Autodesk Inventor part; units mm, degrees
ref_plane "YZ Plane" through (0, 0, 0) normal (1, 0, 0) x (0, 1, 0)
ref_plane "XZ Plane" through (0, 0, 0) normal (0, 1, 0) x (-1, 0, 0)
ref_plane "XY Plane" through (0, 0, 0) normal (0, 0, 1) x (1, 0, 0)
sketch "Sketch1" plane through (0, 0, 0) normal (0, 0, 1) x (1, 0, 0)
  line L0 (-47.5, -14) -> (47.5, -14)
  line L1 (47.5, -14) -> (47.5, 14)
  line L2 (47.5, 14) -> (-47.5, 14)
  line L3 (-47.5, 14) -> (-47.5, -14)
  line L4 (-47.5, -14) -> (47.5, 14) construction
  line L5 (47.5, -14) -> (-47.5, 14) construction
  line L6 (47.5, 14) -> (61.5, 14)
  line L7 (61.5, 14) -> (61.5, -14)
  line L8 (61.5, -14) -> (47.5, -14)
  line L9 (47.5, -14) -> (47.5, 14)
  point P0 (0, 0)
  dimension "d0" = 95
  dimension "d1" = 28
  dimension "d2" = 14
  dimension "d3" = 28
extrude "Extrusion1" add sketch "Sketch1" along normal blind 14
sketch "Sketch2" plane through (0, 0, 14) normal (0, 0, 1) x (1, 0, 0)
  circle A0 centre (47.5, 0) radius 5
  line L0 (61.5, -14) -> (61.5, 14)
  line L1 (-47.5, -14) -> (61.5, -14)
  point P0 (0, 0)
  dimension "d6" = 10
  dimension "d7" = 14
  dimension "d8" = 14
extrude "Extrusion2" cut sketch "Sketch2" against normal blind 14
sketch "Sketch3" plane through (-47.5, -14, 0) normal (-1, 0, 0) x (0, 0, 1)
  circle A0 centre (7, 14) radius 5
  line L0 (0, 28) -> (14, 28)
  line L1 (14, 28) -> (14, 0)
  circle A1 centre (7, 14) radius 25
  point P0 (0, 14)
  dimension "d11" = 10
  dimension "d12" = 14
  dimension "d13" = 7
  dimension "d14" = 50
extrude "Extrusion3" cut sketch "Sketch3" against normal blind 52
properties part number "MSAL Pushing Thing"
Could you check a few things on this model? Use its own coordinates, in mm. Round coordinates to 2 decimals unless told otherwise and drop trailing zeros. Write each loop counter-clockwise with the first axis right and the second up, starting at its lowest first coordinate (ties: lowest second). Pieces come first, ordered by that corner, then holes. Notation, with made-up numbers: (-27, 41.5) -> (-12, 41.5) arc R7 cw to (-12, 50.5) -> close; hole circle Ø9 at (-10.75, 20). An arc over 180 degrees is marked (long way). Use a Markdown table: item, result.
1. If we section it at B-B (x = 47.5): List the corners of the cut face in (y, z) for me.
Answer key:
| item | result |
|---|---|
| outline | (-14, 0) -> (-5, 0) -> (-5, 14) -> (-14, 14) -> close; (5, 0) -> (14, 0) -> (14, 14) -> (5, 14) -> close |
2. If we section it at C-C (y = 0): List the corners of the cut face in (x, z) for me.
Answer key:
| item | result |
|---|---|
| outline | (-47.5, 2) -> (4.5, 2) -> (4.5, 0) -> (42.5, 0) -> (42.5, 14) -> (4.5, 14) -> (4.5, 12) -> (-47.5, 12) -> close; (52.5, 0) -> (61.5, 0) -> (61.5, 14) -> (52.5, 14) -> close |
3. If we section it at A-A (z = 7): List the corners of the cut face in (x, y) for me, then the cut area to 3 significant figures.
Answer key:
| item | result |
|---|---|
| outline | (-47.5, -5) -> (4.5, -5) -> (4.5, -14) -> (61.5, -14) -> (61.5, 14) -> (4.5, 14) -> (4.5, 5) -> (-47.5, 5) -> close; hole circle Ø10 at (47.5, 0) |
| area | 2,040 mm^2 |
4. If we section it at D-D (z = 3): List the corners of the cut face in (x, y) for me.
Answer key:
| item | result |
|---|---|
| outline | (-47.5, -3) -> (4.5, -3) -> (4.5, -14) -> (61.5, -14) -> (61.5, 14) -> (4.5, 14) -> (4.5, 3) -> (-47.5, 3) -> close; hole circle Ø10 at (47.5, 0) |
5. For pin 1 Ø4 at (x, y) = (-29.5, 5.5) entering from +Z; pin 2 Ø9 at (x, y) = (47.5, 0) entering from +Z; pin 3 Ø1.5 at (y, z) = (10.5, 10.5) entering from -X; pin 4 Ø1.5 at (x, z) = (-10, 8) entering from +Y, each with a flat end and sliding along its axis, tell me the tip position at first contact or that it passes through.
Answer key:
| item | result |
|---|---|
| pin 1 | stops at z = 10.57 |
| pin 2 | passes through |
| pin 3 | stops at x = 4.5 |
| pin 4 | stops at y = 4.99 |
6. We'd pull the mould along Y, two halves only. Please class faces 1 (the face through (33, 0, 14)), 2 (the face through (42.505, 0.22, 7.098)), 3 (the face through (33, 14, 7)), 4 (the face through (-21.86, 1.5, 11.77)): +Y half, -Y half, draft (parallel to the pull), parting line (faces both ways), or undercut.
Answer key:
| item | result |
|---|---|
| face 1 | draft |
| face 2 | undercut |
| face 3 | +Y half |
| face 4 | parting line |
7. Please list where these lines run through material, in increasing order: probe 1 along Y at (x, z) = (47.5, 3.5); probe 2 along X at (y, z) = (3.25, 5.5); probe 3 along X at (y, z) = (1, 11.5).
Answer key:
| item | result |
|---|---|
| probe 1 | y = -14 to -5, 5 to 14 |
| probe 2 | x = -47.5 to 43.7, 51.3 to 61.5 |
| probe 3 | x = -47.5 to 42.6, 52.4 to 61.5 |
